Can you work these out from the drawing? Everything is in mm from the part's minimum corner. A direction names the side the tool comes from. Round coordinates to 2 decimals unless told otherwise and drop trailing zeros. Write each loop counter-clockwise with the first axis right and the second up, starting at its lowest first coordinate (ties: lowest second). Pieces come first, ordered by that corner, then holes. Notation, with made-up numbers: M 74,34 L 95,34 A29 ccw 95,66 Z; hole C 41.5,12 d4. An arc over 180 degrees is marked long. Use one line per item in the form item = value. Start each with the question number.
Q1. For the marked faces 4, 5 and 6, which set-ups out of +Z, -Z, +X, -X, +Y, -Y let a thin tool reach every point of the face, with its end or its side?
Q2. I want a section at D-D on z = 2.75. List the corners of the cut face in (x, y) for me.
Q3. I want a section at C-C on x = 5. List the corners of the cut face in (y, z) for me, and give its area (3 significant figures).
Q4. I'm going to push flat-ended pins straight in: pin 1 Ø3.5 at (x, z) = (19, 4) entering from -Y; pin 2 Ø2.5 at (x, z) = (12, 4) entering from -Y; pin 3 Ø2.5 at (x, z) = (6, 3.5) entering from +Y; pin 4 Ø1.8 at (x, z) = (5, 4) entering from -Y. Where does each tip first touch, or does it pass through?
Q5. I want a section at B-B on y = 0.95. List the corners of the cut face in (x, z) for me.
Q6. I want a section at A-A on z = 4. List the corners of the cut face in (x, y) for me, and give its area (3 significant figures).
Q7. We'd pull the mould along Z, two halves only. Please class the marked faces 1, 2 and 3: +Z half, -Z half, draft (parallel to the pull), parting line (faces both ways), or undercut.
Q8. I need wall thicknesses on line 1 along X through (y, z) = (0.65, 4); line 2 along X through (y, z) = (2.3, 6); line 3 along Z through (x, y) = (12, 0.9). Which ranges of each line are inside material? Lowest first, please. Write a range as from..to.
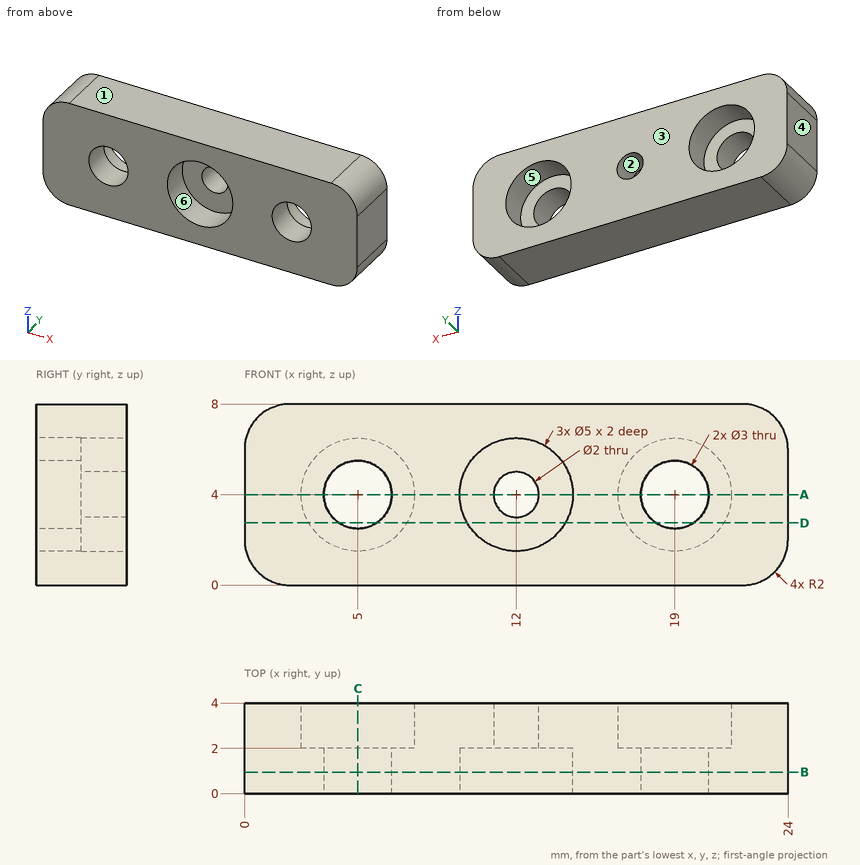
Reported:
q1.face_4 = +Z, -Z, -X, +Y, -Y
q1.face_5 = +Y
q1.face_6 = -Y
q2.outline = M 0,0 L 4.17,0 L 4.17,2 L 2.83,2 L 2.83,4 L 0,4 Z; M 5.83,0 L 9.83,0 L 9.83,2 L 14.17,2 L 14.17,0 L 18.17,0 L 18.17,2 L 16.83,2 L 16.83,4 L 7.17,4 L 7.17,2 L 5.83,2 Z; M 19.83,0 L 24,0 L 24,4 L 21.17,4 L 21.17,2 L 19.83,2 Z
q3.outline = M 0,0 L 4,0 L 4,1.5 L 2,1.5 L 2,2.5 L 0,2.5 Z; M 0,5.5 L 2,5.5 L 2,6.5 L 4,6.5 L 4,8 L 0,8 Z
q3.area = 16.0 mm^2
q4.pin_1 = 0
q4.pin_2 = 2
q4.pin_3 = 2
q4.pin_4 = through
q5.outline = M 0,2 A2 ccw 2,0 L 22,0 A2 ccw 24,2 L 24,6 A2 ccw 22,8 L 2,8 A2 ccw 0,6 Z; hole C 5,4 d3; hole C 12,4 d5; hole C 19,4 d3
q6.outline = M 0,0 L 3.5,0 L 3.5,2 L 2.5,2 L 2.5,4 L 0,4 Z; M 6.5,0 L 9.5,0 L 9.5,2 L 11,2 L 11,4 L 7.5,4 L 7.5,2 L 6.5,2 Z; M 13,2 L 14.5,2 L 14.5,0 L 17.5,0 L 17.5,2 L 16.5,2 L 16.5,4 L 13,4 Z; M 20.5,0 L 24,0 L 24,4 L 21.5,4 L 21.5,2 L 20.5,2 Z
q6.area = 50.0 mm^2
q7.face_1 = +Z half
q7.face_2 = undercut
q7.face_3 = draft
q8.line_1 = 0..3.5, 6.5..9.5, 14.5..17.5, 20.5..24
q8.line_2 = 0..3.5, 6.5..17.5, 20.5..24
q8.line_3 = 0..1.5, 6.5..8
